from build123d import *

# Parameters (mm, degrees)
SKETCH1_R           = 90
BOSS_EXTRUDE2_DEPTH = 5
SKETCH3_W           = 15
SKETCH3_H           = 52
BOSS_EXTRUDE3_DEPTH = 120
CUT_EXTRUDE1_DEPTH  = 80
SKETCH8_R           = 2.1825
SKETCH8_R_2         = 2.18255
CUT_EXTRUDE3_DEPTH  = 80


with BuildPart() as part:
    # Sketch1 → Boss-Extrude2 (new body)
    with BuildSketch(Plane(origin=(0, 0, 0), x_dir=(1, 0, 0), z_dir=(0, 1, 0))):
        with Locations(Location((0, 0, 0), (0, 0, 270))):
            Circle(SKETCH1_R)
    extrude(amount=BOSS_EXTRUDE2_DEPTH)

    # Sketch3 → Boss-Extrude3 (add)
    with BuildSketch(Plane(origin=(0, 0, 0), x_dir=(1, 0, 0), z_dir=(0, 1, 0))):
        Rectangle(SKETCH3_W, SKETCH3_H)
    extrude(amount=BOSS_EXTRUDE3_DEPTH)

    # Sketch5 → Cut-Extrude1 (cut)
    with BuildSketch(Plane.XY.offset(26)):
        Polygon((-5.619057526, 114.98), (-2.720759175, 120), (2.482644122, 120), (5.380942474, 114.98), align=None)
    extrude(amount=-CUT_EXTRUDE1_DEPTH, mode=Mode.SUBTRACT)

    # Sketch8 → Cut-Extrude3 (cut)
    with BuildSketch(Plane.XZ):
        with Locations(Location((26.586875, -75, 0), (0, 0, 270))):
            Circle(SKETCH8_R)
        with Locations(Location((-26.586875, -75, 0), (0, 0, 270))):
            Circle(SKETCH8_R_2)
        with Locations(Location((51.659405284, 60.52328536, 0), (0, 0, 270))):
            Circle(SKETCH8_R)
        with Locations(Location((78.244405284, 14.47671464, 0), (0, 0, 270))):
            Circle(SKETCH8_R)
    extrude(amount=-CUT_EXTRUDE3_DEPTH, mode=Mode.SUBTRACT)


solid = part.part
Design review of the part built by this model. Coordinates are the model's own, in mm. A direction names the side the tool comes from. Give positions to 0.01 mm unless a question says otherwise; leave off trailing zeros. Write each loop counter-clockwise with the first axis right and the second up, starting at its lowest first coordinate (ties: lowest second). Pieces come first, ordered by that corner, then holes. Notation, with made-up numbers: M 46,74.5 L 68,74.5 A5 ccw 68,83.5 Z; hole C 3.5,72.5 d5. An arc over 180 degrees is marked long. Return JSON: item names as keys, results as strings. Group by question number.
Item 1: Clearance check with flat-ended pins moving along their axes: pin 1 Ø1 at (y, z) = (59.5, 11.5) entering from +X; pin 2 Ø7 at (x, z) = (-26.59, -75) entering from +Y; pin 3 Ø10 at (y, z) = (97, 20.5) entering from -X. State where each tip first meets the part, or that it passes through.
Item 2: Take a section at C-C (y = 93.5). Give the boundary of the cut face in (x, z).
Item 3: The part is to be moulded in two halves that separate along X. For faces 1 (the cylindrical face through (80.41, 2.46, 14.76)), 2 (the flat face through (-7.5, 62, 0)), 3 (the flat face through (-19, 5, -1)), say which applies: pulls with the +X half, pulls with the -X half, needs draft (parallel to the pull), parting line crosses it, or undercut.
Item 4: Wall thickness on line 1 along X through (y, z) = (1, -75); line 2 along Y through (x, z) = (43.5, -72); line 3 along X through (y, z) = (35, -22): over which ranges is each line inside the solid? List them lowest first.
Item 5: Tool access review of faces 4 (the flat face through (7.5, 62, 0)), 5 (the flat face through (0, 114.98, 0)), 6 (the flat face through (0, 62, 26)), 7 (the flat face through (0, 62, -26)): name each direction out of +Z, -Z, +X, -X, +Y, -Y from which nothing blocks a thin tool from reaching the whole face with its end or side.
Item 6: Take a section at B-B (z = 0). Give the boundary of the cut face in (x, y).
Item 7: Take a section at D-D (z = 19). Give the boundary of the cut face in (x, y).
Item 8: Take a section at A-A (x = 0). Give the boundary of the cut face in (y, z), plus the area to 3 significant figures.
Return value:
{
 "1": {"pin 1": "stops at x = 7.5", "pin 2": "stops at y = 5", "pin 3": "stops at x = -7.5"},
 "2": {"outline": "M -7.5,-26 L 7.5,-26 L 7.5,26 L -7.5,26 Z"},
 "3": {"face 1": "undercut", "face 2": "pulls with the -X half", "face 3": "needs draft"},
 "4": {"line 1": "x = -49.75 to -28.77, -24.4 to 24.4, 28.77 to 49.75", "line 2": "y = 0 to 5", "line 3": "x = -7.5 to 7.5"},
 "5": {"face 4": "+Z, -Z, +X, +Y", "face 5": "+Z, -Z", "face 6": "+Z, +X, -X, +Y", "face 7": "-Z, +X, -X, +Y"},
 "6": {"outline": "M -90,0 L 90,0 L 90,5 L 7.5,5 L 7.5,120 L 2.48,120 L 5.38,114.98 L -5.62,114.98 L -2.72,120 L -7.5,120 L -7.5,5 L -90,5 Z"},
 "7": {"outline": "M -87.97,0 L 87.97,0 L 87.97,5 L 7.5,5 L 7.5,120 L 2.48,120 L 5.38,114.98 L -5.62,114.98 L -2.72,120 L -7.5,120 L -7.5,5 L -87.97,5 Z"},
 "8": {"outline": "M 0,-90 L 5,-90 L 5,-26 L 114.98,-26 L 114.98,26 L 5,26 L 5,90 L 0,90 Z", "area": "6,620 mm2"}
}
